The drawing under review shows one solid part. Ordinate dimensions are in mm from its lowest x, y, z. A direction names the side the tool comes from. Give positions to 0.01 mm unless a question says otherwise; leave off trailing zeros. Loops run counter-clockwise (first coordinate to the right, second up) from the corner with the lowest first, then second, coordinate; pieces in that order, holes last. Notation, with made-up numbers: (-19.5, 6.25) -> (35.5, 6.25) arc R28 ccw to (35.5, 26.25) -> close; hole circle Ø2 at (22, 41.25). An arc over 180 degrees is marked (long way). Answer in a Markdown table with one row per item. Add a question column.
(1) Consider section A-A on x = 39. Write out the cut boundary in (y, z).
(2) Consider section B-B on y = 68.5. Write out the cut boundary in (x, z), then the cut area to 3 significant figures.
(3) Consider section C-C on z = 41.5. Write out the cut boundary in (x, y).
(4) Consider section D-D on x = 66. Write out the cut boundary in (y, z) (1 decimal), then the cut area to 3 significant figures.
(5) Draft analysis for pull direction Y (two halves, no side actions). For the marked faces 1, 2, 3 and 4, state which applies: +Y half, -Y half, draft (parallel to the pull), parting line (faces both ways), or undercut.
(6) For line 1 (Y direction, x = 45.5, z = 67); line 2 (Y direction, x = 67, z = 83); line 3 (Y direction, x = 47, z = 52), list the stretches that pass through material, from the lowest coordinate up.
(7) For pin 1 (12 mm diameter, centred on y = 47, z = 36, fed in from -X); pin 2 (4 mm diameter, centred on x = 28, y = 35.5, fed in from +Z); pin 3 (4 mm diameter, centred on x = 35.5, z = 76.5, fed in from +Y), all flat-tipped, find the tip position at first contact; note any pin that passes through.
(8) For the marked faces 5, 6 and 7, list the 3-axis set-ups (+Z, -Z, +X, -X, +Y, -Y) from which the entire face can be reached by the end or side of a thin tool; tool diameter is ignored.
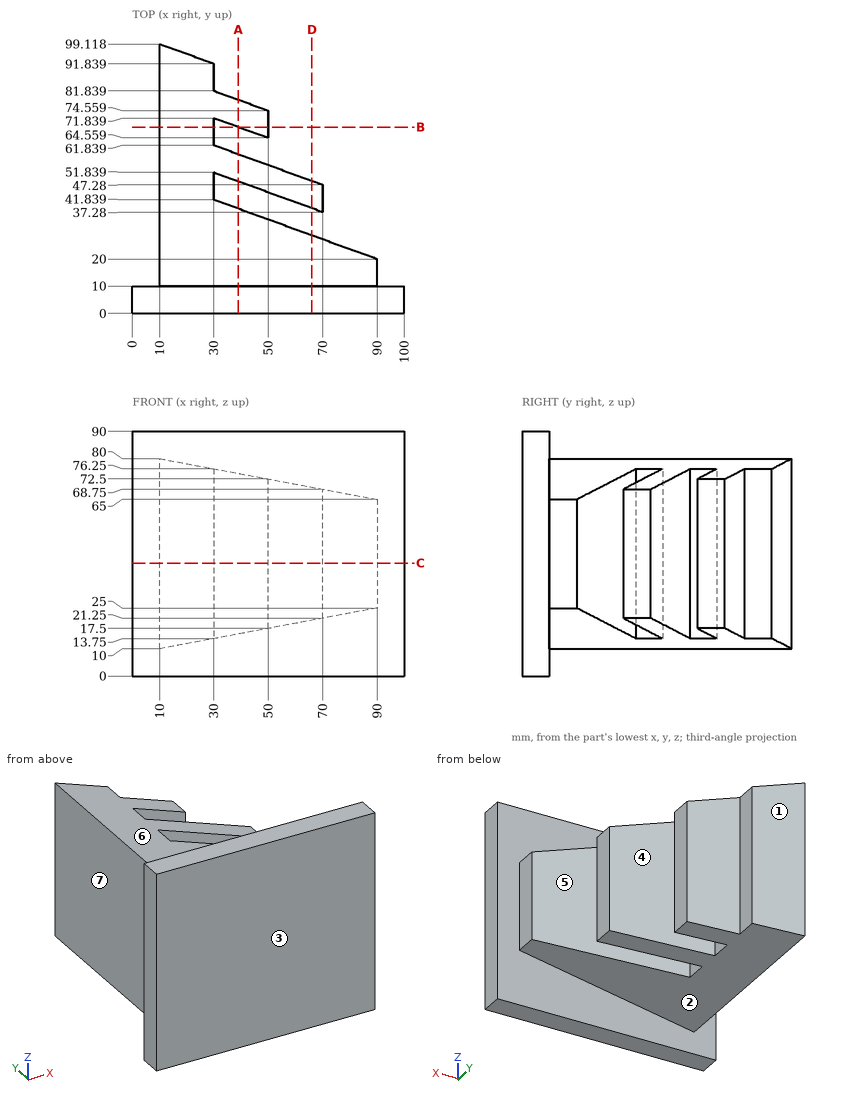
Values follow:
| question | item | result |
|---|---|---|
| 1 | outline | (0, 0) -> (10, 0) -> (10, 15.44) -> (38.56, 15.44) -> (38.56, 74.56) -> (10, 74.56) -> (10, 90) -> (0, 90) -> close; (48.56, 15.44) -> (58.56, 15.44) -> (58.56, 74.56) -> (48.56, 74.56) -> close; (68.56, 15.44) -> (78.56, 15.44) -> (78.56, 74.56) -> (68.56, 74.56) -> close |
| 2 | outline | (10, 10) -> (30, 13.75) -> (30, 76.25) -> (10, 80) -> close; (39.17, 15.47) -> (50, 17.5) -> (50, 72.5) -> (39.17, 74.53) -> close |
| 2 | area | 1,940 mm2 |
| 3 | outline | (0, 0) -> (100, 0) -> (100, 10) -> (90, 10) -> (90, 20) -> (30, 41.84) -> (30, 51.84) -> (70, 37.28) -> (70, 47.28) -> (30, 61.84) -> (30, 71.84) -> (50, 64.56) -> (50, 74.56) -> (30, 81.84) -> (30, 91.84) -> (10, 99.12) -> (10, 10) -> (0, 10) -> close |
| 4 | outline | (0, 0) -> (10, 0) -> (10, 20.5) -> (28.7, 20.5) -> (28.7, 69.5) -> (10, 69.5) -> (10, 90) -> (0, 90) -> close; (38.7, 20.5) -> (48.7, 20.5) -> (48.7, 69.5) -> (38.7, 69.5) -> close |
| 4 | area | 2,310 mm2 |
| 5 | face 1 | +Y half |
| 5 | face 2 | draft |
| 5 | face 3 | -Y half |
| 5 | face 4 | undercut |
| 6 | line 1 | 0 to 36.2, 46.2 to 56.2, 66.2 to 76.2 |
| 6 | line 2 | 0 to 10 |
| 6 | line 3 | 0 to 35.65, 45.65 to 55.65, 65.65 to 75.65 |
| 7 | pin 1 | x = 10 |
| 7 | pin 2 | z = 77 |
| 7 | pin 3 | y = 80.48 |
| 8 | face 5 | +Z, -Z |
| 8 | face 6 | +Z, +X, +Y |
| 8 | face 7 | +Z, -Z, -X, +Y |
